```python
from build123d import *

# Parameters (mm, degrees)
F1_DEPTH = 10
F2_DEPTH = 7


with BuildPart() as f1:
    # F0 (on Front) → F1 (new body)
    with BuildSketch(Plane.XZ):
        with BuildLine():
            ThreePointArc((0, 34.5), (-10.606602, 30.106602), (-15, 19.5))
            Line((-15, 19.5), (0, 19.5))
            Line((0, 19.5), (15, 19.5))
            ThreePointArc((15, 19.5), (10.606602, 30.106602), (0, 34.5))
        make_face()
        with BuildLine():
            ThreePointArc((-18, 19.5), (-12.727922, 6.772078), (0, 1.5))
            ThreePointArc((0, 1.5), (12.727922, 6.772078), (18, 19.5))
            Line((18, 19.5), (15, 19.5))
            ThreePointArc((15, 19.5), (0, 4.5), (-15, 19.5))
            Line((-15, 19.5), (-18, 19.5))
        make_face()
        Polygon((0, 1.5), (-18, 1.5), (-18, -1.5), (18, -1.5), (18, 1.5), align=None)
        with BuildLine():
            ThreePointArc((18, 19.5), (12.727922, 6.772078), (0, 1.5))
            Line((0, 1.5), (18, 1.5))
            Line((18, 1.5), (18, 19.5))
        make_face()
        with BuildLine():
            Line((0, 19.5), (-15, 19.5))
            ThreePointArc((-15, 19.5), (0, 4.5), (15, 19.5))
            Line((15, 19.5), (0, 19.5))
        make_face()
        with BuildLine():
            Line((15, 19.5), (18, 19.5))
            ThreePointArc((18, 19.5), (12.727922, 32.227922), (0, 37.5))
            Line((0, 37.5), (0, 34.5))
            ThreePointArc((0, 34.5), (10.606602, 30.106602), (15, 19.5))
        make_face()
        with BuildLine():
            ThreePointArc((0, 37.5), (-12.727922, 32.227922), (-18, 19.5))
            Line((-18, 19.5), (-15, 19.5))
            ThreePointArc((-15, 19.5), (-10.606602, 30.106602), (0, 34.5))
            Line((0, 34.5), (0, 37.5))
        make_face()
        with BuildLine():
            Line((-18, 19.5), (-18, 1.5))
            Line((-18, 1.5), (0, 1.5))
            ThreePointArc((0, 1.5), (-12.727922, 6.772078), (-18, 19.5))
        make_face()
    extrude(amount=F1_DEPTH)

    # F0 (on Front) → F2 (cut)
    with BuildSketch(Plane.XZ):
        with BuildLine():
            Line((0, 19.5), (-15, 19.5))
            ThreePointArc((-15, 19.5), (0, 4.5), (15, 19.5))
            Line((15, 19.5), (0, 19.5))
        make_face()
        with BuildLine():
            ThreePointArc((0, 34.5), (-10.606602, 30.106602), (-15, 19.5))
            Line((-15, 19.5), (0, 19.5))
            Line((0, 19.5), (15, 19.5))
            ThreePointArc((15, 19.5), (10.606602, 30.106602), (0, 34.5))
        make_face()
    extrude(amount=F2_DEPTH, mode=Mode.SUBTRACT)


solid = f1.part
```
Design review of the part built by this model. Coordinates are the model's own, in mm. Give positions to 0.01 mm unless a question says otherwise; leave off trailing zeros. Order: outer loops, then holes, each group sorted by start corner. A loop starts at its lowest first (then second) coordinate and runs counter-clockwise, first axis right, second up. Notation, with made-up numbers: (37.25, 6.25) -> (68.25, 6.25) arc R15 cw to (68.25, 11.25) -> close; hole circle Ø7 at (58.5, -22). An arc over 180 degrees is marked (long way). Write item = value, one per line. Start each with the question number.
(1) To check wall thickness, follow line 1 along X through (y, z) = (-5.75, 19.5); line 2 along Y through (x, z) = (1.5, 27); line 3 along Z through (x, y) = (-4, -1.5). State the ranges of each line that lie inside material, in increasing order.
(2) We need section C-C on x = -6.5. Write out the cut boundary in (y, z), plus the area to 3 significant figures.
(3) We need section A-A on y = -4.5. Write out the cut boundary in (x, z), plus the area to 3 significant figures.
(4) For pin 1 (1 mm diameter, centred on x = -4.5, z = 8.5, fed in from +Y); pin 2 (1 mm diameter, centred on x = -4.5, y = -6.5, fed in from +Z); pin 3 (6 mm diameter, centred on x = 11, y = -1, fed in from +Z), all flat-tipped, find the tip position at first contact; note any pin that passes through.
(5) Mouldability with a two-part tool opening along X and no side actions: class faces 1 (the face through (-18, -5, 9)), 2 (the face through (0, -7, 20)), 3 (the face through (18, -5, 9)), 4 (the face through (8, 0, 5)) as +X half, -X half, draft (parallel to the pull), parting line (faces both ways), or undercut.
(6) We need section B-B on z = 14. Write out the cut boundary in (x, y), plus the area to 3 significant figures.
Numbers:
q1.line_1 = -18 to -15, 15 to 18
q1.line_2 = -10 to -7
q1.line_3 = -1.5 to 5.04, 33.96 to 37.05
q2.outline = (-10, -1.5) -> (0, -1.5) -> (0, 5.98) -> (-7, 5.98) -> (-7, 33.02) -> (0, 33.02) -> (0, 36.29) -> (-10, 36.29) -> close
q2.area = 189 mm^2
q3.outline = (-18, -1.5) -> (18, -1.5) -> (18, 19.5) arc R18 ccw to (-18, 19.5) -> close; hole (0, 34.5) arc R15 ccw (long way) to (15, 19.5) arc R15 ccw to start
q3.area = 558 mm^2
q4.pin_1 = -7
q4.pin_2 = 37.05
q4.pin_3 = 35.62
q5.face_1 = -X half
q5.face_2 = undercut
q5.face_3 = +X half
q5.face_4 = draft
q6.outline = (-18, -10) -> (18, -10) -> (18, 0) -> (13.96, 0) -> (13.96, -7) -> (-13.96, -7) -> (-13.96, 0) -> (-18, 0) -> close
q6.area = 165 mm^2
